The listing builds one solid part. Answer for the finished solid, in the listing's coordinates (mm). A direction names the side the tool comes from. Give positions to 0.01 mm unless a question says otherwise; leave off trailing zeros. Loops run counter-clockwise (first coordinate to the right, second up) from the corner with the lowest first, then second, coordinate; pieces in that order, holes last. Notation, with made-up numbers: M -3,57 L 7,57 A21 cw 7,91 Z; hole C -22.75,28.5 d6. An arc over 180 degrees is marked long. One line per item, written item: value. Start each with the question number.
Q1. A cutting plane is placed at C-C, the plane y = 27. Determine the outline of the cut face in (x, z), and give its area (3 significant figures).
Q2. A cutting plane is placed at B-B, the plane z = 1.65. State how many separate pieces and enclosed holes the cut face has, and give its area (3 significant figures).
Q3. The mould has two halves that part along X. Classify faces 1 (the cylindrical face through (-45.872, 15.371, 1.521)), 2 (the cylindrical face through (45.6, 15.6, 1.5)), 3 (the cylindrical face through (-100.914, -14.939, 1.479)): +X half, -X half, draft (parallel to the pull), parting line (faces both ways), or undercut.
Q4. For faces 4 (the cylindrical face through (-0.627, 44.996, 1.479)), 5 (the flat face through (63.66, -58.84, 1.48)), determine the directions among +Z, -Z, +X, -X, +Y, -Y from which every point of the face is accessible in a straight line to the end or side of a thin tool.
Q5. A cutting plane is placed at A-A, the plane x = 0. Determine the outline of the cut face in (y, z).
Q6. A cutting plane is placed at D-D, the plane x = 28. Determine the outline of the cut face in (y, z), and give its area (3 significant figures).
Q7. A flat-ended cylindrical pin translates along its axis: pin 1 (5 mm diameter, centred on x = 43.56, y = -45.1, fed in from +Z). Find the tip coordinate at first contact, or state that the pin passes through.
Q8. Consider L1, parallel to Y at x = 0, z = 2; L2, parallel to X at y = -58, z = 1.95; L3, parallel to Y at x = 94, z = 1.4. Determine where each line is inside the solid, lowest interval first.
from build123d import *

# Parameters (mm, degrees)
SKETCH1_R           = 20
SKETCH1_R_2         = 2.1
BOSS_EXTRUDE1_DEPTH = 3
FILLET1_R           = 40


with BuildPart() as part:
    # Sketch1 → Boss-Extrude1 (new body)
    with BuildSketch(Plane.XY):
        with BuildLine():
            Line((-93.417721196, -71.166653094), (-116.378727138, -15.733881143))
            Line((-116.378727138, -15.733881143), (-42.468364537, 14.880793446))
            ThreePointArc((-42.468364537, 14.880793446), (0, 45), (42.468364537, 14.880793446))
            Line((42.468364537, 14.880793446), (116.378727138, -15.733881143))
            Line((116.378727138, -15.733881143), (93.417721196, -71.166653094))
            Line((93.417721196, -71.166653094), (19.507358595, -40.551978505))
            ThreePointArc((19.507358595, -40.551978505), (0, -45), (-19.507358595, -40.551978505))
            Line((-19.507358595, -40.551978505), (-93.417721196, -71.166653094))
        make_face()
        Circle(SKETCH1_R, mode=Mode.SUBTRACT)
        with Locations((-93.34973001, -38.666724214)):
            Circle(SKETCH1_R_2, mode=Mode.SUBTRACT)
        with Locations((-102.916815819, -15.569735901)):
            Circle(SKETCH1_R_2, mode=Mode.SUBTRACT)
        with Locations((-84.838757104, -59.214030433)):
            Circle(SKETCH1_R_2, mode=Mode.SUBTRACT)
        with Locations((84.838757104, -59.214030433)):
            Circle(SKETCH1_R_2, mode=Mode.SUBTRACT)
        with Locations((93.34973001, -38.666724214)):
            Circle(SKETCH1_R_2, mode=Mode.SUBTRACT)
        with Locations((102.916815819, -15.569735901)):
            Circle(SKETCH1_R_2, mode=Mode.SUBTRACT)
        with Locations((-62.691100974, 1.092300744)):
            Circle(SKETCH1_R_2, mode=Mode.SUBTRACT)
        with Locations((-53.124015165, -22.004687569)):
            Circle(SKETCH1_R_2, mode=Mode.SUBTRACT)
        with Locations((-43.556929356, -45.101675882)):
            Circle(SKETCH1_R_2, mode=Mode.SUBTRACT)
        with Locations((43.556929356, -45.101675882)):
            Circle(SKETCH1_R_2, mode=Mode.SUBTRACT)
        with Locations((53.124015165, -22.004687569)):
            Circle(SKETCH1_R_2, mode=Mode.SUBTRACT)
        with Locations((62.691100974, 1.092300744)):
            Circle(SKETCH1_R_2, mode=Mode.SUBTRACT)
    extrude(amount=BOSS_EXTRUDE1_DEPTH)

    # Fillet1
    fillet1_edges = [part.edges().sort_by_distance(p)[0] for p in [
        (-19.507358595, -40.551978505, 1.5),
        (-42.468364537, 14.880793446, 1.5),
        (42.468364537, 14.880793446, 1.5),
        (19.507358595, -40.551978505, 1.5),
    ]]
    fillet(fillet1_edges, radius=FILLET1_R)


solid = part.part
Answer block:
1. outline: M -36,0 L 36,0 L 36,3 L -36,3 Z
1. area: 216 mm^2
2. separate pieces: 1
2. enclosed holes: 13
2. area: 13,700 mm^2
3. face 1: -X half
3. face 2: +X half
3. face 3: undercut
4. face 4: +Z, -Z, +Y
4. face 5: +Z, -Z, -Y
5. outline: M -45,0 L -20,0 L -20,3 L -45,3 Z; M 20,0 L 45,0 L 45,3 L 20,3 Z
6. outline: M -44.46,0 L 35.23,0 L 35.23,3 L -44.46,3 Z
6. area: 239 mm^2
7. pin 1: z = 3
8. L1: -45 to -20, 20 to 45
8. L2: -98.87 to -86.55, -83.13 to -61.63, 61.63 to 83.13, 86.55 to 98.87
8. L3: -69.76 to -40.66, -36.67 to -6.46
